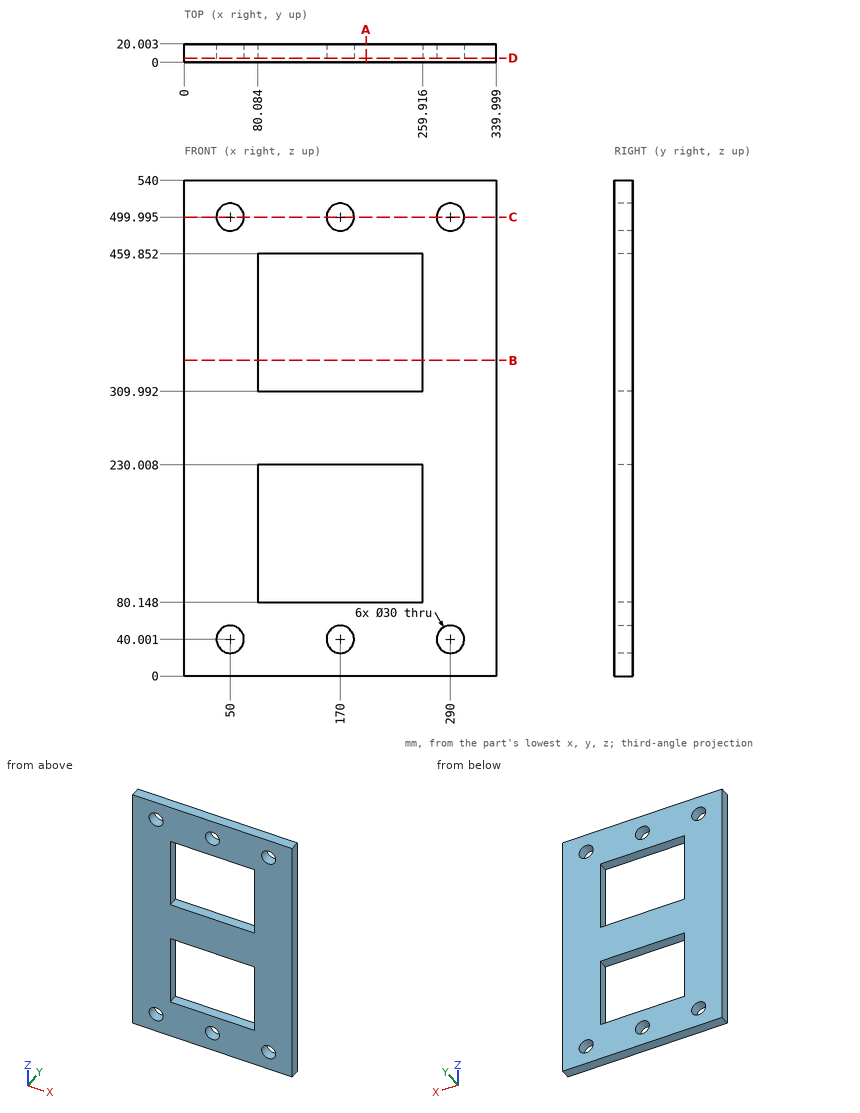
Part print with two shaded views. Sizes in mm from the minimum x, y, z corner. Give positions to 0.01 mm unless a question says otherwise; leave off trailing zeros. Write each loop counter-clockwise with the first axis right and the second up, starting at its lowest first coordinate (ties: lowest second). Pieces come first, ordered by that corner, then holes.
1) Cut at D-D on y = 4.5. State how many separate pieces and enclosed holes the cut face has, then the cut area to 3 significant figures.
Resolved:
separate pieces: 1
enclosed holes: 8
area: 125,000 mm2
2) Cut at A-A on x = 198. Write the cut outline in (y, z), then the cut area to 3 significant figures.
Resolved:
outline: (0, 0) - (20, 0) - (20, 80.15) - (0, 80.15) - close; (0, 230.01) - (20, 230.01) - (20, 309.99) - (0, 309.99) - close; (0, 459.85) - (20, 459.85) - (20, 540) - (0, 540) - close
area: 4,810 mm2
3) Probe L1, parallel to Z at x = 201, y = 1.25; L2, parallel to X at y = 4, z = 129.5 (1 decimal); L3, parallel to Z at x = 301.5, y = 15.25 (1 decimal). List the from-to ranges inside material, lowest first.
Resolved:
L1: z = 0 to 80.15, 230.01 to 309.99, 459.85 to 540
L2: x = 0 to 80.1, 259.9 to 340
L3: z = 0 to 30.4, 49.6 to 490.4, 509.6 to 540
4) Cut at B-B on z = 344. Write the cut outline in (x, y) (1 decimal), then the cut area to 3 significant figures.
Resolved:
outline: (0, 0) - (80.1, 0) - (80.1, 20) - (0, 20) - close; (259.9, 0) - (340, 0) - (340, 20) - (259.9, 20) - close
area: 3,200 mm2
5) Cut at C-C on z = 500. Write the cut outline in (x, y).
Resolved:
outline: (0, 0) - (35, 0) - (35, 20) - (0, 20) - close; (65, 0) - (155, 0) - (155, 20) - (65, 20) - close; (185, 0) - (275, 0) - (275, 20) - (185, 20) - close; (305, 0) - (340, 0) - (340, 20) - (305, 20) - close
